```python
from build123d import *

# Parameters (mm, degrees)
EXTRUDE_1_DEPTH = 125
FILLET_1_R      = 30


with BuildPart() as part:
    # ｽｹｯﾁ1 → ﾎﾞｽ - 押し出し1 (new body)
    with BuildSketch(Plane.XY):
        with BuildLine():
            Line((-101, 0), (-101, 33.466401061))
            ThreePointArc((-101, 33.466401061), (-78.978867604, 53.677045675), (-50, 61))
            Line((-50, 61), (0, 61))
            Line((0, 61), (0, 66))
            Line((0, 66), (-50, 66))
            ThreePointArc((-50, 66), (-82.02123597, 57.711701127), (-106, 34.928498393))
            Line((-106, 34.928498393), (-106, 0))
            Line((-106, 0), (-101, 0))
        make_face()
    extrude(amount=EXTRUDE_1_DEPTH)

    # ﾌｨﾚｯﾄ1
    fillet_1_edges = [part.edges().sort_by_distance(p)[0] for p in [
        (-106, 34.928498393, 62.5),
    ]]
    fillet(fillet_1_edges, radius=FILLET_1_R)


solid = part.part
```
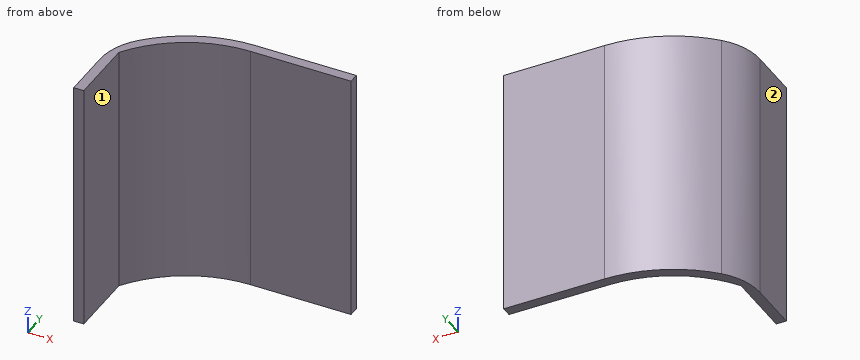
For this review, take the finished solid that the model builds, in its own axes (mm). Face numbers are marked on the shaded views. A direction names the side the tool comes from. Coordinates: 2 decimals unless noted, no trailing zeros. Loops run counter-clockwise (first coordinate to the right, second up) from the corner with the lowest first, then second, coordinate; pieces in that order, holes last. Notation, with made-up numbers: (72, -2) - (95, -2) arc R27 cw to (95, 14) - close; hole circle Ø3 at (-10.75, -16). An arc over 180 degrees is marked (long way). Use one line per item in the form item = value. Start each with the question number.
1) For the marked faces 1 and 2, list the 3-axis set-ups (+Z, -Z, +X, -X, +Y, -Y) from which the entire face can be reached by the end or side of a thin tool; tool diameter is ignored.
2) To check wall thickness, follow probe 1 along X at (y, z) = (8, 28.5); probe 2 along Y at (x, z) = (-51.5, 82); probe 3 along X at (y, z) = (31.5, 77.5). State the ranges of each line that lie inside material, in increasing order. Write a range as from..to.
3) Take a section at A-A (z = 86). State the section outline as (x, y) points.
4) For pin 1 (1 mm diameter, centred on y = 31.5, z = 90.5, fed in from +X); pin 2 (10 mm diameter, centred on x = -82.5, z = 88, fed in from +Y); pin 3 (6 mm diameter, centred on y = 59, z = 64.5, fed in from +X); pin 4 (3 mm diameter, centred on y = 45.5, z = 19, fed in from +X), all flat-tipped, find the tip position at first contact; note any pin that passes through.
5) Take a section at C-C (y = 20.5). State the section outline as (x, z) points, plus the area to 3 significant figures.
6) Take a section at B-B (x = -43.5). State the section outline as (y, z) points, plus the area to 3 significant figures.
From the geometry:
q1.face_1 = +Z, -Z, +X, -Y
q1.face_2 = +Z, -Z, -X, +Y, -Y
q2.probe_1 = -106..-101
q2.probe_2 = 60.98..65.98
q2.probe_3 = -105.26..-101
q3.outline = (-106, 0) - (-101, 0) - (-101, 33.47) arc R61 cw to (-50, 61) - (0, 61) - (0, 66) - (-50, 66) arc R66 ccw to (-97.67, 45.65) arc R30 ccw to (-106, 24.9) - close
q4.pin_1 = -101
q4.pin_2 = 60
q4.pin_3 = 0
q4.pin_4 = -88.88
q5.outline = (-106, 0) - (-101, 0) - (-101, 125) - (-106, 125) - close
q5.area = 625 mm2
q6.outline = (61, 0) - (66, 0) - (66, 125) - (61, 125) - close
q6.area = 625 mm2
